Read the model definition and answer for the solid it produces. Units are mm, in the model's axes. A direction names the side the tool comes from. Round coordinates to 2 decimals unless told otherwise and drop trailing zeros. Write each loop counter-clockwise with the first axis right and the second up, starting at its lowest first coordinate (ties: lowest second). Pieces come first, ordered by that corner, then holes. Notation, with made-up numbers: (73, 25) - (94, 25) arc R22 cw to (94, 63) - close; hole circle Ø9 at (41, -8). An arc over 180 degrees is marked (long way). One line per item, written item: value. Start each with the question number.
(1) Flat-ended cylindrical pins translate along their axes: pin 1 Ø2 at (x, y) = (5, 8.5) entering from -Z; pin 2 Ø2 at (y, z) = (5.5, -3) entering from +X. Find the tip coordinate at first contact, or state that the pin passes through.
(2) A cutting plane is placed at C-C, the plane x = 5.25. Determine the outline of the cut face in (y, z), plus the area to 3 significant figures.
(3) A cutting plane is placed at A-A, the plane z = 0. Determine the outline of the cut face in (x, y).
(4) A cutting plane is placed at B-B, the plane y = 0.75. Determine the outline of the cut face in (x, z).
(5) Find the intervals of material crossed by L1, parallel to Z at x = 0, y = 4.75; L2, parallel to Z at x = 0, y = 3.5; L3, parallel to X at y = 1.5, z = 0, in increasing order.
(6) For faces 1 (the face through (2.492, 1.479, -4.335)), 2 (the face through (-3, 3, -1)), 3 (the face through (5.69, 1.48, 0.75)), determine the directions among +Z, -Z, +X, -X, +Y, -Y from which every point of the face is accessible in a straight line to the end or side of a thin tool.
(7) A cutting plane is placed at D-D, the plane x = -3.25. Determine the outline of the cut face in (y, z).
(8) The mould has two halves that part along Y. Classify faces 4 (the face through (3, 4, -1)), 5 (the face through (3, 9.5, -1)), 6 (the face through (-2.196, 1.479, 5.303)): +Y half, -Y half, draft (parallel to the pull), parting line (faces both ways), or undercut.
Autodesk Inventor part; units mm, degrees
ref_plane "YZ Plane" through (0, 0, 0) normal (1, 0, 0) x (0, 1, 0)
ref_plane "XZ Plane" through (0, 0, 0) normal (0, 1, 0) x (-1, 0, 0)
ref_plane "XY Plane" through (0, 0, 0) normal (0, 0, 1) x (1, 0, 0)
sketch "Sketch1" plane through (0, 0, 0) normal (0, 1, 0) x (-1, 0, 0)
  circle A0 centre (0, 0) radius 6.5
  arc A1 (4.9572, -0.6526) -> (4.9572, 0.6526) centre (0, 0) ccw
  line L0 (6.5, 0) -> (0, 0)
  line L1 (4.9572, -0.6526) -> (6.4979, -0.8555)
  line L2 (4.9572, 0.6526) -> (6.9401, 0.9137)
  line L3 (0, 0) -> (7, 0) construction
  line L4 (3.0438, 3.9668) -> (3.9898, 5.1996)
  arc A2 (3.0438, 3.9668) -> (1.9134, 4.6194) centre (0, 0) ccw
  line L5 (1.9134, 4.6194) -> (2.6788, 6.4672)
  line L6 (-1.9134, 4.6194) -> (-2.5081, 6.0551)
  arc A3 (-1.9134, 4.6194) -> (-3.0438, 3.9668) centre (0, 0) ccw
  line L7 (-3.0438, 3.9668) -> (-4.2613, 5.5535)
  line L8 (-4.9572, 0.6526) -> (-6.4979, 0.8555)
  arc A4 (-4.9572, 0.6526) -> (-4.9572, -0.6526) centre (0, 0) ccw
  line L9 (-4.9572, -0.6526) -> (-6.9401, -0.9137)
  line L10 (-3.0438, -3.9668) -> (-3.9898, -5.1996)
  arc A5 (-3.0438, -3.9668) -> (-1.9134, -4.6194) centre (0, 0) ccw
  line L11 (-1.9134, -4.6194) -> (-2.6788, -6.4672)
  line L12 (1.9134, -4.6194) -> (2.5081, -6.0551)
  arc A6 (1.9134, -4.6194) -> (3.0438, -3.9668) centre (0, 0) ccw
  line L13 (3.0438, -3.9668) -> (4.2613, -5.5535)
  point P0 (-6.4444, -0.8484)
  point P1 (-3.9569, -5.1568)
  point P2 (-2.4874, -6.0052)
  point P3 (2.4874, -6.0052)
  point P4 (3.9569, -5.1568)
  point P5 (6.4444, -0.8484)
  point P6 (6.4444, 0.8484)
  point P7 (3.9569, 5.1568)
  point P8 (2.4874, 6.0052)
  point P9 (-2.4874, 6.0052)
  point P10 (-3.9569, 5.1568)
  point P11 (-6.4444, 0.8484)
  dimension "d0" = 13
  dimension "d1" = 10
  dimension "d2" = 6.554
  dimension "d3" = 7.5
  dimension "d4" = 7
  dimension "d5" = 7.5
  dimension "d8" = 360
extrude "Extrusion1" add sketch "Sketch1" along normal blind 3 contours L2 A1 L1 A0 L13 A6 L12 L11 A5 L10 L9 A4 L8 L7 A3 L6 L5 A2 L4
sketch "Sketch2" plane through (0, 3, 0) normal (0, 1, 0) x (1, 0, 0)
  arc A0 (-2.4874, -6.0052) -> (2.4874, -6.0052) centre (0, 0) ccw
  line L0 (2.4874, -6.0052) -> (1.9134, -4.6194)
  arc A1 (1.9134, -4.6194) -> (3.0438, -3.9668) centre (0, 0) ccw
  line L1 (3.0438, -3.9668) -> (3.9569, -5.1568)
  arc A2 (3.9569, -5.1568) -> (6.4444, -0.8484) centre (0, 0) ccw
  line L2 (6.4444, -0.8484) -> (4.9572, -0.6526)
  arc A3 (4.9572, -0.6526) -> (4.9572, 0.6526) centre (0, 0) ccw
  line L3 (4.9572, 0.6526) -> (6.4444, 0.8484)
  arc A4 (6.4444, 0.8484) -> (3.9569, 5.1568) centre (0, 0) ccw
  line L4 (3.9569, 5.1568) -> (3.0438, 3.9668)
  arc A5 (3.0438, 3.9668) -> (1.9134, 4.6194) centre (0, 0) ccw
  line L5 (1.9134, 4.6194) -> (2.4874, 6.0052)
  arc A6 (2.4874, 6.0052) -> (-2.4874, 6.0052) centre (0, 0) ccw
  line L6 (-2.4874, 6.0052) -> (-1.9134, 4.6194)
  arc A7 (-1.9134, 4.6194) -> (-3.0438, 3.9668) centre (0, 0) ccw
  line L7 (-3.0438, 3.9668) -> (-3.9569, 5.1568)
  arc A8 (-3.9569, 5.1568) -> (-6.4444, 0.8484) centre (0, 0) ccw
  line L8 (-6.4444, 0.8484) -> (-4.9572, 0.6526)
  arc A9 (-4.9572, 0.6526) -> (-4.9572, -0.6526) centre (0, 0) ccw
  line L9 (-4.9572, -0.6526) -> (-6.4444, -0.8484)
  arc A10 (-6.4444, -0.8484) -> (-3.9569, -5.1568) centre (0, 0) ccw
  line L10 (-3.9569, -5.1568) -> (-3.0438, -3.9668)
  arc A11 (-3.0438, -3.9668) -> (-1.9134, -4.6194) centre (0, 0) ccw
  line L11 (-1.9134, -4.6194) -> (-2.4874, -6.0052)
  circle A12 centre (0, 0) radius 3
  dimension "d12" = 6
extrude "Extrusion2" add sketch "Sketch2" along normal blind 1 contours A12
sketch "Sketch3" plane through (0, 4, 0) normal (0, 1, 0) x (1, 0, 0)
  circle A0 centre (0, 0) radius 3.5
  dimension "d15" = 7
extrude "Extrusion3" add sketch "Sketch3" along normal blind 5.5
sketch "Sketch4" plane through (0, 9.5, 0) normal (0, 1, 0) x (1, 0, 0)
  point P0 (0, 0)
  point P1 (0, 0)
hole "Hole1" at (0, 9.5, 0) direction (0, -1, 0) diameter 4 end through all countersink diameter 6 countersink angle 90
thread "Thread1"
properties material "Brass, Soft Yellow, Welded"
Here are the results:
1. pin 1: through
1. pin 2: x = 2.87
2. outline: (0, -3.83) - (3, -3.83) - (3, -0.69) - (0, -0.69) - close; (0, 0.69) - (3, 0.69) - (3, 3.83) - (0, 3.83) - close
2. area: 18.8 mm²
3. outline: (-5, 0) - (-2, 0) - (-2, 8.5) - (-3, 9.5) - (-3.5, 9.5) - (-3.5, 4) - (-3, 4) - (-3, 3) - (-5, 3) - close; (2, 0) - (5, 0) - (5, 3) - (3, 3) - (3, 4) - (3.5, 4) - (3.5, 9.5) - (3, 9.5) - (2, 8.5) - close
4. outline: (-6.44, -0.85) arc R6.5 ccw to (-3.96, -5.16) - (-3.04, -3.97) arc R5 ccw to (-1.91, -4.62) - (-2.49, -6.01) arc R6.5 ccw to (2.49, -6.01) - (1.91, -4.62) arc R5 ccw to (3.04, -3.97) - (3.96, -5.16) arc R6.5 ccw to (6.44, -0.85) - (4.96, -0.65) arc R5 ccw to (4.96, 0.65) - (6.44, 0.85) arc R6.5 ccw to (3.96, 5.16) - (3.04, 3.97) arc R5 ccw to (1.91, 4.62) - (2.49, 6.01) arc R6.5 ccw to (-2.49, 6.01) - (-1.91, 4.62) arc R5 ccw to (-3.04, 3.97) - (-3.96, 5.16) arc R6.5 ccw to (-6.44, 0.85) - (-4.96, 0.65) arc R5 ccw to (-4.96, -0.65) - close; hole circle Ø4 at (0, 0)
5. L1: -3.5 to -2, 2 to 3.5
5. L2: -3 to -2, 2 to 3
5. L3: -5 to -2, 2 to 5
6. face 1: +Y, -Y
6. face 2: none
6. face 3: +X, +Y, -Y
7. outline: (0, -4.24) - (3, -4.24) - (3, 4.24) - (0, 4.24) - close; (4, -1.3) - (9.5, -1.3) - (9.5, 1.3) - (4, 1.3) - close
8. face 4: undercut
8. face 5: +Y half
8. face 6: draft
